```python
from build123d import *

# Parameters (mm, degrees)
F1_DEPTH = 7.5
F2_W     = 10
F2_H     = 10
F3_DEPTH = 20.001


with BuildPart() as f1:
    # F0 (on Front) → F1 (new body, symmetric)
    with BuildSketch(Plane.XZ):
        Polygon((0, 20), (0, 0), (5, 0), (5, 2.5), (20, 2.5), (20, 0), (30, 0), (30, 7.5), (14.5, 20), align=None)
    extrude(amount=F1_DEPTH, both=True)

    # F2 (on face) → F3 (cut, through all)
    with BuildSketch(Plane.XY.offset(20)):
        with Locations((25, 0)):
            Rectangle(F2_W, F2_H)
    extrude(amount=-F3_DEPTH, mode=Mode.SUBTRACT)


solid = f1.part
```
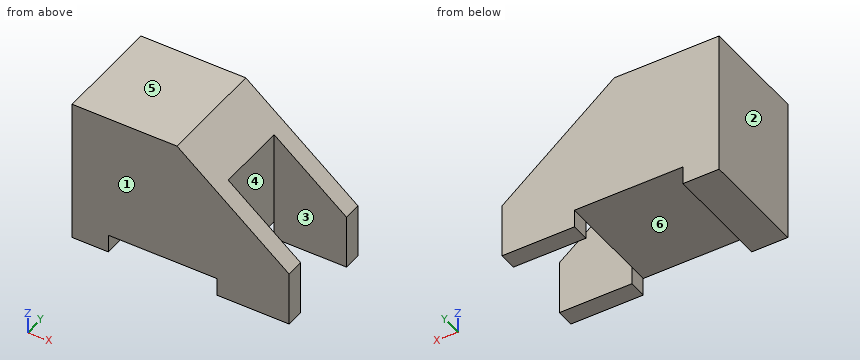
Here's how the part is built. I have some questions about the finished solid (model axes, mm). Face numbers are marked on the shaded views. A direction names the side the tool comes from. Coordinates: 2 decimals unless noted, no trailing zeros. Order: outer loops, then holes, each group sorted by start corner. A loop starts at its lowest first (then second) coordinate and runs counter-clockwise, first axis right, second up.
1) Imagine slicing it at A-A on z = 15.25. List the corners of the cut face in (x, y) for me.
2) Which directions (+Z, -Z, +X, -X, +Y, -Y) give clear straight access to the entire face, cutting with the end or side of a thin tool? Please do the marked faces 4, 5 and 6.
3) We'd pull the mould along Y, two halves only. Please class the marked faces 1, 2 and 3: +Y half, -Y half, draft (parallel to the pull), parting line (faces both ways), or undercut.
4) Will these pins go through, and if not, where does the flat tip stop? pin 1 (0.8 mm diameter, centred on y = 0.5, z = 2, fed in from +X); pin 2 (7.5 mm diameter, centred on x = 11, y = 3, fed in from -Z); pin 3 (3 mm diameter, centred on y = -5.5, z = 1.5, fed in from -X).
5) Imagine slicing it at C-C on x = 24.25. List the corners of the cut face in (y, z) for me, and give its area (3 significant figures).
6) Imagine slicing it at B-B on y = -2. List the corners of the cut face in (x, z) for me, and give its area (3 significant figures).
7) I need wall thicknesses on line 1 (X direction, y = 4.25, z = 5.25); line 2 (X direction, y = -6, z = 1.25); line 3 (Z direction, x = 8.5, y = -0.5). Which ranges of each line are inside material? Lowest first, please.
8) Imagine slicing it at D-D on x = 9.5. List the corners of the cut face in (y, z) for me.
Response values:
1. outline: (0, -7.5) - (20.39, -7.5) - (20.39, -5) - (20, -5) - (20, 5) - (20.39, 5) - (20.39, 7.5) - (0, 7.5) - close
2. face 4: +Z, -Z, +X
2. face 5: +Z, +X, -X, +Y, -Y
2. face 6: -Z, +Y, -Y
3. face 1: -Y half
3. face 2: draft
3. face 3: undercut
4. pin 1: stops at x = 5
4. pin 2: stops at z = 2.5
4. pin 3: stops at x = 0
5. outline: (-7.5, 0) - (-5, 0) - (-5, 12.14) - (-7.5, 12.14) - close; (5, 0) - (7.5, 0) - (7.5, 12.14) - (5, 12.14) - close
5. area: 60.7 mm2
6. outline: (0, 0) - (5, 0) - (5, 2.5) - (20, 2.5) - (20, 15.56) - (14.5, 20) - (0, 20) - close
6. area: 350 mm2
7. line 1: x = 0 to 20
7. line 2: x = 0 to 5, 20 to 30
7. line 3: z = 2.5 to 20
8. outline: (-7.5, 2.5) - (7.5, 2.5) - (7.5, 20) - (-7.5, 20) - close
